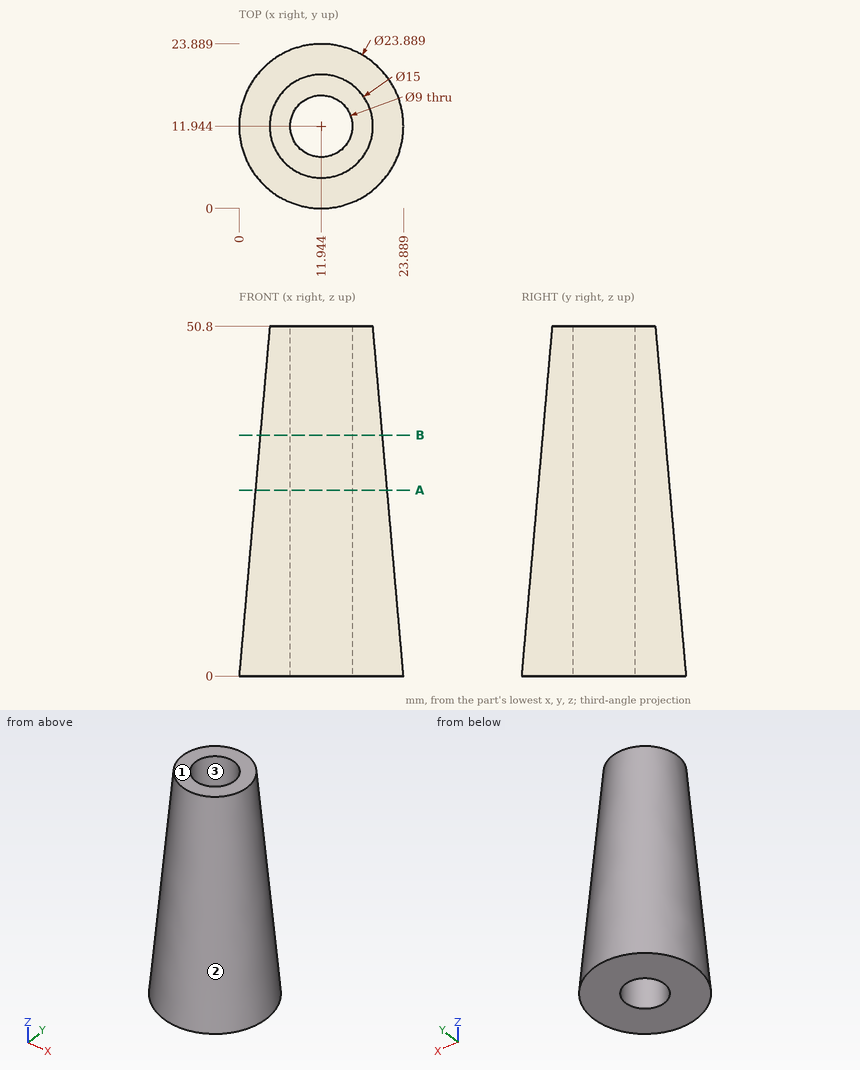
Verification items for this drawing (mm, ordinates from the low corner). Coordinates: 2 decimals unless noted, no trailing zeros. Loops run counter-clockwise (first coordinate to the right, second up) from the corner with the lowest first, then second, coordinate; pieces in that order, holes last. Notation, with made-up numbers: (-18.75, 23) -> (-0.75, 23) arc R33 cw to (-0.75, 57) -> close; hole circle Ø9 at (32.5, 7.25). An arc over 180 degrees is marked (long way). Put each result on its own line as item: value.
1. Mould release check, pull along X, two halves, no side actions. Record for the marked faces 1, 2 and 3: pulls with the +X half, pulls with the -X half, needs draft (parallel to the pull), parting line crosses it, or undercut.
Result set:
face 1: needs draft
face 2: parting line crosses it
face 3: undercut
2. Thickness scan on line 1 (Y direction, x = 13, z = 41) (1 decimal); line 2 (X direction, y = 9, z = 41.5); line 3 (Y direction, x = 13, z = 36.5). Record the ranges inside material, lowest first.
Result set:
line 1: y = 3.7 to 7.6, 16.3 to 20.2
line 2: x = 4.17 to 8.54, 15.35 to 19.72
line 3: y = 3.26 to 7.57, 16.32 to 20.63
3. Gauge pin test, flat ends, axial feed: P1, Ø8, axis at x = 15, z = 15.5, coming from the -Y side; P2, Ø8, axis at x = 2.5, z = 27, coming from the -Y side; P3, Ø4, axis at y = 21, z = 7.5, coming from the +X side. Record the tip position at first contact, or that the pin passes through.
Result set:
P1: stops at y = 1.1
P2: stops at y = 4.03
P3: stops at x = 20.77
4. Section check B-B, the plane z = 35. Record the boundary of the cut face in (x, y) (1 decimal).
Result set:
outline: circle Ø17.8 at (11.9, 11.9); hole circle Ø9 at (11.9, 11.9)
5. Section check A-A, the plane z = 27. Record the boundary of the cut face in (x, y) (1 decimal).
Result set:
outline: circle Ø19.2 at (11.9, 11.9); hole circle Ø9 at (11.9, 11.9)
